For this review, take the finished solid that the model builds, in its own axes (mm). Round coordinates to 2 decimals unless told otherwise and drop trailing zeros. Order: outer loops, then holes, each group sorted by start corner. A loop starts at its lowest first (then second) coordinate and runs counter-clockwise, first axis right, second up. Notation, with made-up numbers: M -34,47.25 L 10,47.25 A25 ccw 10,64.25 Z; hole C 44.5,-13 d9. An arc over 180 degrees is marked long. Use a Markdown table: item, result.
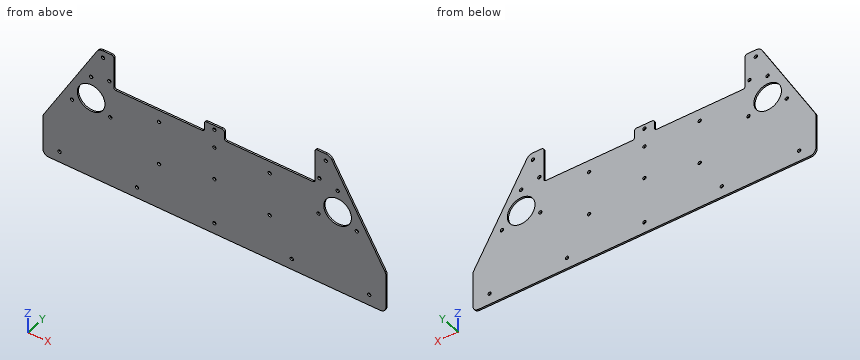
from build123d import *

# Parameters (mm, degrees)
ESQUISSE1_R             = 1.5
ESQUISSE1_R_2           = 12.5
BOSS_EXTRU_1_DEPTH      = 1.5
CONG_2_R                = 5
ESQUISSE2_R             = 1.5
ESQUISSE2_W             = 182
ESQUISSE2_H             = 32
ENL_V_MAT_EXTRU_1_DEPTH = 223.771744169
ESQUISSE3_W             = 18
ESQUISSE3_H             = 10
BOSS_EXTRU_2_DEPTH      = 1.5
CONG_3_R                = 2
ESQUISSE4_R             = 1.5
ENL_V_MAT_EXTRU_2_DEPTH = 3


with BuildPart() as part:
    # Esquisse1 → Boss.-Extru.1 (new body)
    with BuildSketch(Plane(origin=(0, 0, 0), x_dir=(1, 0, 0), z_dir=(0, 1, 0))):
        with BuildLine():
            Line((-155, -35), (155, -35))
            Line((155, -35), (155, -72.562177826))
            Line((155, -72.562177826), (106.394138206, -156.75))
            ThreePointArc((106.394138206, -156.75), (104.014973081, -159.129165125), (100.764973081, -160))
            Line((100.764973081, -160), (-100.764973081, -160))
            ThreePointArc((-100.764973081, -160), (-104.014973081, -159.129165125), (-106.394138206, -156.75))
            Line((-106.394138206, -156.75), (-155, -72.562177826))
            Line((-155, -72.562177826), (-155, -35))
        make_face()
        with Locations(Location((-70, -45, 0), (0, 0, 270))):
            Circle(ESQUISSE1_R, mode=Mode.SUBTRACT)
        with Locations(Location((0, -45, 0), (0, 0, 270))):
            Circle(ESQUISSE1_R, mode=Mode.SUBTRACT)
        with Locations(Location((111.445953061, -110, 0), (0, 0, 270))):
            Circle(ESQUISSE1_R_2, mode=Mode.SUBTRACT)
        with Locations(Location((128.766461137, -100, 0), (0, 0, 270))):
            Circle(ESQUISSE1_R, mode=Mode.SUBTRACT)
        with Locations(Location((94.125444985, -100, 0), (0, 0, 270))):
            Circle(ESQUISSE1_R, mode=Mode.SUBTRACT)
        with Locations(Location((111.445953061, -130, 0), (0, 0, 270))):
            Circle(ESQUISSE1_R, mode=Mode.SUBTRACT)
        with Locations(Location((70, -45, 0), (0, 0, 90))):
            Circle(ESQUISSE1_R, mode=Mode.SUBTRACT)
        with Locations(Location((-140, -45, 0), (0, 0, 270))):
            Circle(ESQUISSE1_R, mode=Mode.SUBTRACT)
        with Locations(Location((140, -45, 0), (0, 0, 90))):
            Circle(ESQUISSE1_R, mode=Mode.SUBTRACT)
        with Locations(Location((-100.764973081, -153.5, 0), (0, 0, 270))):
            Circle(ESQUISSE1_R, mode=Mode.SUBTRACT)
        with Locations(Location((100.764973081, -153.5, 0), (0, 0, 90))):
            Circle(ESQUISSE1_R, mode=Mode.SUBTRACT)
        with Locations(Location((-111.445953061, -130, 0), (0, 0, 90))):
            Circle(ESQUISSE1_R, mode=Mode.SUBTRACT)
        with Locations(Location((-128.766461137, -100, 0), (0, 0, 90))):
            Circle(ESQUISSE1_R, mode=Mode.SUBTRACT)
        with Locations(Location((-111.445953061, -110, 0), (0, 0, 90))):
            Circle(ESQUISSE1_R_2, mode=Mode.SUBTRACT)
        with Locations(Location((-94.125444985, -100, 0), (0, 0, 90))):
            Circle(ESQUISSE1_R, mode=Mode.SUBTRACT)
    extrude(amount=BOSS_EXTRU_1_DEPTH)

    # Congé2
    cong_2_edges = [part.edges().sort_by_distance(p)[0] for p in [
        (-155, 0.75, 35),
        (155, 0.75, 35),
        (155, 0.75, 72.562177826),
        (-155, 0.75, 72.562177826),
    ]]
    fillet(cong_2_edges, radius=CONG_2_R)

    # Esquisse2 → Enlèv. mat.-Extru.1 (cut, through all)
    with BuildSketch(Plane(origin=(0, 1.5, 0), x_dir=(1, 0, 0), z_dir=(0, 1, 0))):
        with Locations(Location((-50, -77, 0), (0, 0, 270))):
            Circle(ESQUISSE2_R)
        with Locations(Location((-50, -117, 0), (0, 0, 270))):
            Circle(ESQUISSE2_R)
        with Locations(Location((50, -117, 0), (0, 0, 90))):
            Circle(ESQUISSE2_R)
        with Locations(Location((50, -77, 0), (0, 0, 90))):
            Circle(ESQUISSE2_R)
        with Locations(Location((0, -117, 0), (0, 0, 270))):
            Circle(ESQUISSE2_R)
        with Locations(Location((0, -87, 0), (0, 0, 270))):
            Circle(ESQUISSE2_R)
        with Locations((0, -144)):
            Rectangle(ESQUISSE2_W, ESQUISSE2_H)
    extrude(amount=-ENL_V_MAT_EXTRU_1_DEPTH, mode=Mode.SUBTRACT)

    # Esquisse3 → Boss.-Extru.2 (add)
    with BuildSketch(Plane(origin=(0, 1.5, 0), x_dir=(1, 0, 0), z_dir=(0, 1, 0))):
        with Locations((0, -133)):
            Rectangle(ESQUISSE3_W, ESQUISSE3_H)
    extrude(amount=-BOSS_EXTRU_2_DEPTH)

    # Congé3
    cong_3_edges = [part.edges().sort_by_distance(p)[0] for p in [
        (-91, 0.75, 160),
        (-91, 0.75, 128),
        (91, 0.75, 128),
        (91, 0.75, 160),
        (-9, 0.75, 138),
        (-9, 0.75, 128),
        (9, 0.75, 128),
        (9, 0.75, 138),
    ]]
    fillet(cong_3_edges, radius=CONG_3_R)

    # Esquisse4 → Enlèv. mat.-Extru.2 (cut)
    with BuildSketch(Plane(origin=(0, 1.5, 0), x_dir=(1, 0, 0), z_dir=(0, 1, 0))):
        with Locations(Location((-95, -134, 0), (0, 0, 270))):
            Circle(ESQUISSE4_R)
        with Locations(Location((0, -134, 0), (0, 0, 270))):
            Circle(ESQUISSE4_R)
        with Locations(Location((95, -134, 0), (0, 0, 270))):
            Circle(ESQUISSE4_R)
    extrude(amount=-ENL_V_MAT_EXTRU_2_DEPTH, mode=Mode.SUBTRACT)


solid = part.part
Q1. Clearance check with a flat-ended pin moving along its axis: pin 1 (0.8 mm diameter, centred on y = 0.5, z = 137.5, fed in from +X). State where the tip first meets the part, or that it passes through.
Determined:
| item | result |
|---|---|
| pin 1 | stops at x = 117.74 |
Q2. Wall thickness on line 1 along X through (y, z) = (0.8, 120.5); line 2 along X through (y, z) = (1.25, 153.5); line 3 along X through (y, z) = (1.2, 105.5): over which ranges is each line inside the solid? List them lowest first. Write a range as [from, to].
Determined:
| item | result |
|---|---|
| line 1 | x = [-127.32, -118.23], [-104.66, 104.66], [118.23, 127.32] |
| line 2 | x = [-108.27, -102.26], [-99.26, -91], [91, 99.26], [102.26, 108.27] |
| line 3 | x = [-135.98, -123.11], [-99.78, 99.78], [123.11, 135.98] |
Q3. Add section A-A (z = 107). Write out the cut boundary in (x, y), then the cut area to 3 significant figures.
Determined:
| item | result |
|---|---|
| outline | M -135.12,0 L -123.58,0 L -123.58,1.5 L -135.12,1.5 Z; M -99.31,0 L 99.31,0 L 99.31,1.5 L -99.31,1.5 Z; M 123.58,0 L 135.12,0 L 135.12,1.5 L 123.58,1.5 Z |
| area | 333 mm^2 |
Q4. Add section B-B (z = 145.5). Write out the cut boundary in (x, y).
Determined:
| item | result |
|---|---|
| outline | M -112.89,0 L -91,0 L -91,1.5 L -112.89,1.5 Z; M 91,0 L 112.89,0 L 112.89,1.5 L 91,1.5 Z |
Q5. Add section C-C (x = -86). Write out the cut boundary in (y, z), then the cut area to 4 significant figures.
Determined:
| item | result |
|---|---|
| outline | M 0,35 L 1.5,35 L 1.5,128 L 0,128 Z |
| area | 139.5 mm^2 |
